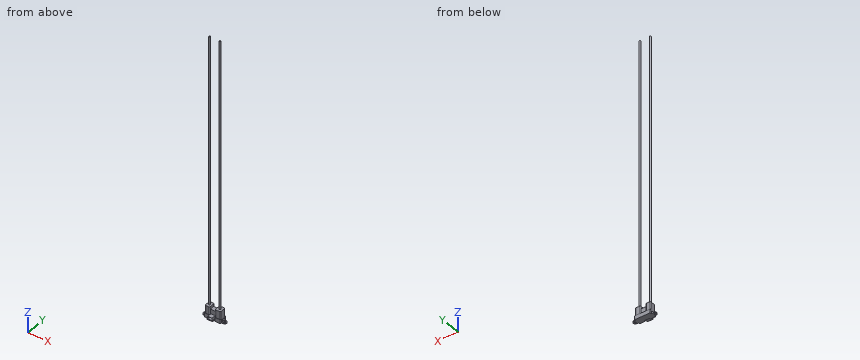
```python
from build123d import *

# Parameters (mm, degrees)
EXTRUDE_1_DEPTH     = 7.2
SKETCH_2_R          = 1.6
EXTRUDE_2_DEPTH     = 1.5
EXTRUDE_START       = -7.5
EXTRUDE_3_DEPTH     = 7.5
EXTRUDE_4_DEPTH     = 10.1
SKETCH_7_R          = 3.75
CUT_EXTRUDE_3_DEPTH = 21.5
SKETCH_8_W          = 10.45
SKETCH_8_H          = 11.9
EXTRUDE_5_DEPTH     = 14.4
FILLET_1_R          = 1.75
EXTRUDE_6_DEPTH     = 9.9
SKETCH_10_W         = 8.1
SKETCH_10_H         = 8.2
EXTRUDE_7_DEPTH     = 5
SKETCH_11_W         = 7.7
SKETCH_11_H         = 4.6
CUT_EXTRUDE_4_DEPTH = 8.2
SKETCH_13_R         = 1.5
EXTRUDE_9_DEPTH     = 500


with BuildPart() as part:
    # 草图1 → 凸台-拉伸1 (new body)
    with BuildSketch(Plane.XY):
        Polygon((14.75, -6.5), (4.675, -6.5), (4.675, -4.2), (-5.425, -4.2), (-5.425, -6.5), (-14.75, -6.5), (-14.75, 6.5), (14.75, 6.5), align=None)
    extrude(amount=EXTRUDE_1_DEPTH)

    # 草图2 → 凸台-拉伸2 (add)
    # profile 1 of 2: a face of its own
    with BuildSketch(Plane.XY):
        with BuildLine():
            Line((-18.5, 3.75), (-14.75, 3.75))
            Line((-14.75, 3.75), (-14.75, -3.75))
            Line((-14.75, -3.75), (-18.5, -3.75))
            ThreePointArc((-18.5, -3.75), (-22.25, 0), (-18.5, 3.75))
        make_face()
        with Locations((-18.5, 0)):
            Circle(SKETCH_2_R, mode=Mode.SUBTRACT)
    # profile 2 of 2: a face of its own
    with BuildSketch(Plane.XY):
        with BuildLine():
            Line((18.5, 3.75), (14.75, 3.75))
            Line((14.75, 3.75), (14.75, 0))
            Line((14.75, 0), (14.75, -3.75))
            Line((14.75, -3.75), (18.5, -3.75))
            ThreePointArc((18.5, -3.75), (22.25, 0), (18.5, 3.75))
        make_face()
        with Locations((18.5, 0)):
            Circle(SKETCH_2_R, mode=Mode.SUBTRACT)
    extrude(amount=EXTRUDE_2_DEPTH)

    # 草图3 → 凸台-拉伸3 (add)
    with BuildSketch(Plane(origin=(0, 3.75, 0), x_dir=(1, 0, 0), z_dir=(0, 1, 0)).offset(EXTRUDE_START)):
        Polygon((-14.75, -1.5), (-14.75, -5.5), (-17.578427125, -2.671572875), (-18.012250402, -1.5), align=None)
    extrude_3 = extrude(amount=EXTRUDE_3_DEPTH)

    # 草图5 → 凸台-拉伸4 (add)
    with BuildSketch(Plane(origin=(-5.425, 0, 0), x_dir=(0, 0, -1), z_dir=(1, 0, 0))):
        Polygon((-3.9, -4.2), (-2.7, -4.2), (-2.7, -6.5), (-2.7, -12.4), (-3.9, -12.4), align=None)
    extrude(amount=EXTRUDE_4_DEPTH)

    # 草图7 → 切除-拉伸3 (cut)
    with BuildSketch(Plane.XY.offset(1.5)):
        with Locations((-18.5, 0)):
            Circle(SKETCH_7_R)
        with BuildLine():
            Line((-18.012250402, 1.523843932), (-18.012250402, -1.523843932))
            ThreePointArc((-18.012250402, -1.523843932), (-20.1, 0), (-18.012250402, 1.523843932))
        make_face(mode=Mode.SUBTRACT)
    cut_extrude_3 = extrude(amount=CUT_EXTRUDE_3_DEPTH, mode=Mode.SUBTRACT)

    # 镜向2: 凸台-拉伸3, 切除-拉伸3 across plane
    add(extrude_3.mirror(Plane(origin=(0, 0, 0), x_dir=(0, 0, 1), z_dir=(1, 0, 0))))
    add(cut_extrude_3.mirror(Plane(origin=(0, 0, 0), x_dir=(0, 0, 1), z_dir=(1, 0, 0))), mode=Mode.SUBTRACT)

    # 草图8 → 凸台-拉伸5 (add)
    with BuildSketch(Plane.XY.offset(7.2)):
        Polygon((-14.75, 0), (-14.75, 5.95), (-5.8, 5.95), (-5.8, -5.95), (-14.75, -5.95), align=None)
        with Locations((9.525, 0)):
            Rectangle(SKETCH_8_W, SKETCH_8_H)
    extrude(amount=EXTRUDE_5_DEPTH)

    # 圆角1
    # the kernel refuses this fillet: 1.75 mm, written as the material it takes off along each edge
    with BuildSketch(Plane(origin=(-14.75, -5.95, 7.2), x_dir=(0, 1, 0), z_dir=(0, 0, 1)), Plane(origin=(14.75, 5.95, 7.2), x_dir=(0, -1, 0), z_dir=(0, 0, 1))) as fillet_1_piece_1:
        with BuildLine():
            CenterArc((FILLET_1_R, -FILLET_1_R), FILLET_1_R, 90, 90)
            Line((0, -FILLET_1_R), (0, 0))
            Line((0, 0), (FILLET_1_R, 0))
        make_face()
    extrude(amount=18.775, mode=Mode.SUBTRACT)
    with BuildSketch(Plane(origin=(-5.8, -5.95, 7.2), x_dir=(0, 1, 0), z_dir=(0, 0, 1)), Plane(origin=(-5.8, 5.95, 7.2), x_dir=(-1, 0, 0), z_dir=(0, 0, 1)), Plane(origin=(-14.75, 5.95, 7.2), x_dir=(0, -1, 0), z_dir=(0, 0, 1)), Plane(origin=(14.75, -5.95, 7.2), x_dir=(0, 1, 0), z_dir=(0, 0, 1)), Plane(origin=(4.3, 5.95, 7.2), x_dir=(0, -1, 0), z_dir=(0, 0, 1)), Plane(origin=(4.3, -5.95, 7.2), x_dir=(1, 0, 0), z_dir=(0, 0, 1))) as fillet_1_piece_2:
        with BuildLine():
            CenterArc((FILLET_1_R, FILLET_1_R), FILLET_1_R, 180, 90)
            Line((0, FILLET_1_R), (0, 0))
            Line((0, 0), (FILLET_1_R, 0))
        make_face()
    extrude(amount=18.775, mode=Mode.SUBTRACT)

    # 草图9 → 凸台-拉伸6 (add)
    with BuildSketch(Plane.XY.offset(7.2)):
        Polygon((-5.8, 0), (-5.8, 4.2), (4.3, 4.2), (4.3, -4.2), (-5.8, -4.2), align=None)
    extrude(amount=EXTRUDE_6_DEPTH)

    # 草图10 → 凸台-拉伸7 (add)
    with BuildSketch(Plane.XY.offset(3.9)):
        with Locations((-0.375, -8.3)):
            Rectangle(SKETCH_10_W, SKETCH_10_H)
    extrude(amount=EXTRUDE_7_DEPTH)

    # 草图11 → 切除-拉伸4 (cut)
    with BuildSketch(Plane.XZ.offset(12.4)):
        with Locations((-0.375, 6.4)):
            Rectangle(SKETCH_11_W, SKETCH_11_H)
    extrude(amount=-CUT_EXTRUDE_4_DEPTH, mode=Mode.SUBTRACT)

    # 草图13 → 凸台-拉伸9 (add)
    with BuildSketch(Plane.XY.offset(21.6)):
        with Locations((-10.275, 0)):
            Circle(SKETCH_13_R)
        with Locations((9.525, 0)):
            Circle(SKETCH_13_R)
    extrude(amount=EXTRUDE_9_DEPTH)


solid = part.part
```
CAD build for the part. Positions are in the model's coordinates, mm. Round coordinates to 2 decimals unless told otherwise and drop trailing zeros. Order: outer loops, then holes, each group sorted by start corner. A loop starts at its lowest first (then second) coordinate and runs counter-clockwise, first axis right, second up. Notation, with made-up numbers: (36, -14.5) - (50, -14.5) arc R27 cw to (50, 19.5) - close; hole circle Ø7 at (-2.5, -4.5). An arc over 180 degrees is marked (long way). Answer as CSV lines item,"result". Start each with the question number.
1. Pin check, flat tips, straight feed: pin 1 (2 mm diameter, centred on x = -9.5, z = 2.5, fed in from -Y); pin 2 (2 mm diameter, centred on x = -3.5, y = -4.5, fed in from +Z); pin 3 (8.5 mm diameter, centred on x = 7.5, y = 1, fed in from +Z); pin 4 (2.5 mm diameter, centred on x = -1, z = 7, fed in from -Y). Stop position of each tip, or through.
2. Saw through at A-A, the plane z = 306. Write the cut outline in (x, y) (3 decimals).
3. Drill centre lines: L1, parallel to Z at x = 0.5, y = -5; L2, parallel to Y at x = -18.5, z = 0.55. Where is each one in solid material? Low to high. Write a range as [from, to].
Model answer:
1,pin 1,"stops at y = -6.5"
1,pin 2,"stops at z = 17.1"
1,pin 3,"stops at z = 521.6"
1,pin 4,"stops at y = -4.2"
2,outline,"circle Ø3 at (-10.275, 0); circle Ø3 at (9.525, 0)"
3,L1,"z = [2.7, 4.1], [8.7, 8.9]"
3,L2,"y = [-3.75, -1.6], [1.6, 3.75]"
